Verification items for the finished model (mm, model axes). Face numbers are marked on the shaded views. A direction names the side the tool comes from. Round coordinates to 2 decimals unless told otherwise and drop trailing zeros. Write each loop counter-clockwise with the first axis right and the second up, starting at its lowest first coordinate (ties: lowest second). Pieces come first, ordered by that corner, then holes. Notation, with made-up numbers: M 56,-9 L 74,-9 A24 ccw 74,12 Z; hole C 58,14.5 d10. An arc over 180 degrees is marked long. One line per item, written item: value. Start each with the question number.
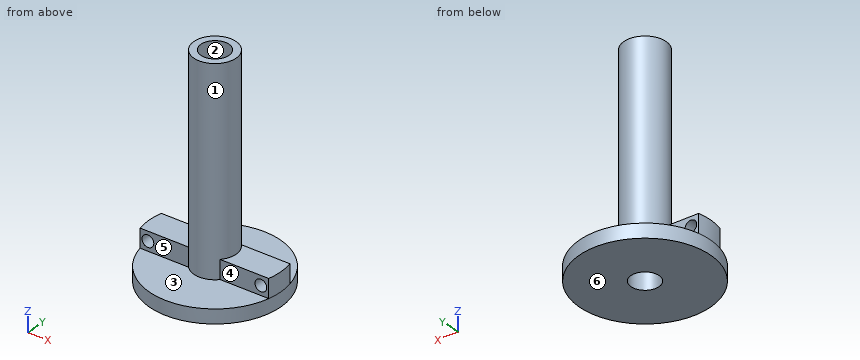
from build123d import *
from build123d.topology import SkipClean

# Parameters (mm, degrees)
SKETCH1_R           = 7
BOSS_EXTRUDE1_DEPTH = 1.5
SKETCH2_R           = 2.25
BOSS_EXTRUDE2_DEPTH = 21.5
CUT_EXTRUDE1_REACH  = 27.04
SKETCH4_R           = 1.5
BOSS_EXTRUDE5_DEPTH = 2
CUT_EXTRUDE5_REACH  = 27.5
SKETCH16_R          = 0.625
CUT_EXTRUDE6_REACH  = 25.67
SKETCH17_R          = 1.5


with BuildPart() as part:
    # Sketch1 → Boss-Extrude1 (new body)
    with BuildSketch(Plane.XY):
        Circle(SKETCH1_R)
    extrude(amount=BOSS_EXTRUDE1_DEPTH)

    # Sketch2 → Boss-Extrude2 (add)
    with BuildSketch(Plane.XY.offset(1.5)):
        Circle(SKETCH2_R)
    extrude(amount=BOSS_EXTRUDE2_DEPTH)

    # Sketch4 → Cut-Extrude1 (cut, up to next)
    with BuildSketch(Plane(origin=(0, 0, 0), x_dir=(-1, 0, 0), z_dir=(0, 0, -1)), mode=Mode.PRIVATE) as cut_extrude1_sk1:
        Circle(SKETCH4_R)
    cut_extrude1_tool1 = extrude(cut_extrude1_sk1.sketch, amount=-CUT_EXTRUDE1_REACH, mode=Mode.PRIVATE) & part.part
    add(cut_extrude1_tool1.solids().sort_by_distance((0, 0, 0))[0], mode=Mode.SUBTRACT)

    # Sketch15 → Boss-Extrude5 (add)
    with SkipClean():  # the faces are left unmerged after this step: merging them gives an invalid solid
        with BuildSketch(Plane.XY.offset(1.5)):
            with BuildLine():
                Line((6.837397, -1.5), (-6.837397, -1.5))
                ThreePointArc((-6.837397, -1.5), (-7, 0), (-6.837397, 1.5))
                Line((-6.837397, 1.5), (6.837397, 1.5))
                ThreePointArc((6.837397, 1.5), (7, 0), (6.837397, -1.5))
            make_face()
        extrude(amount=BOSS_EXTRUDE5_DEPTH)

    # Sketch16 → Cut-Extrude5 (cut, up to next)
    with BuildSketch(Plane.XZ.offset(1.5), mode=Mode.PRIVATE) as cut_extrude5_sk1:
        with Locations((-6, 2.5)):
            Circle(SKETCH16_R)
    cut_extrude5_tool1 = extrude(cut_extrude5_sk1.sketch, amount=-CUT_EXTRUDE5_REACH, mode=Mode.PRIVATE) & part.part
    # Sketch16 → Cut-Extrude5 (cut, up to next)
    with BuildSketch(Plane.XZ.offset(1.5), mode=Mode.PRIVATE) as cut_extrude5_sk2:
        with Locations(Location((6, 2.5, 0), (0, 0, 270))):
            Circle(SKETCH16_R)
    cut_extrude5_tool2 = extrude(cut_extrude5_sk2.sketch, amount=-CUT_EXTRUDE5_REACH, mode=Mode.PRIVATE) & part.part
    add(cut_extrude5_tool1.solids().sort_by_distance((-6, -1.5, 2.5))[0], mode=Mode.SUBTRACT)
    add(cut_extrude5_tool2.solids().sort_by_distance((6, -1.5, 2.5))[0], mode=Mode.SUBTRACT)

    # Sketch17 → Cut-Extrude6 (cut, up to next)
    with BuildSketch(Plane(origin=(0, 0, 1.5), x_dir=(-1, 0, 0), z_dir=(0, 0, -1)), mode=Mode.PRIVATE) as cut_extrude6_sk1:
        Circle(SKETCH17_R)
    cut_extrude6_tool1 = extrude(cut_extrude6_sk1.sketch, amount=-CUT_EXTRUDE6_REACH, mode=Mode.PRIVATE) & part.part
    add(cut_extrude6_tool1.solids().sort_by_distance((0, 0, 1.5))[0], mode=Mode.SUBTRACT)


solid = part.part
1) Thickness scan on line 1 (X direction, y = -0.5, z = 2) (3 decimals); line 2 (Y direction, x = 0, z = 14); line 3 (Z direction, x = -6, y = -0.9) (3 decimals). Record the ranges inside material, lowest first.
2) Mould release check, pull along X, two halves, no side actions. Record for the marked faces 1, 2 and 3: pulls with the +X half, pulls with the -X half, needs draft (parallel to the pull), parting line crosses it, or undercut.
3) Cross-section at D-D (z = 12.75). Record the boundary of the cut face in (x, y).
4) Gauge pin test, flat ends, axial feed: pin 1 Ø1.1 at (x, z) = (-6, 2.5) entering from -Y; pin 2 Ø1.6 at (x, z) = (3.5, 2) entering from +Y; pin 3 Ø1.5 at (x, y) = (-2.5, -5.5) entering from -Z; pin 4 Ø3.5 at (x, y) = (-5, 0) entering from +Z. Record the tip position at first contact, or that the pin passes through.
5) Cross-section at C-C (x = 0). Record the boundary of the cut face in (y, z).
6) Cross-section at B-B (z = 2.5). Record the boundary of the cut face in (x, y) (3 decimals), then the cut area to 3 significant figures.
7) Cross-section at A-A (y = 0). Record the boundary of the cut face in (x, z) (3 decimals), then the cut area to 3 significant figures.
8) Access from +Z, -Z, +X, -X, +Y, -Y to the whole of each face (thin tool, end or side, straight path). Record for the marked faces 4, 5 and 6.
Results below:
1. line 1: x = -6.982 to -6.375, -5.625 to -1.414, 1.414 to 5.625, 6.375 to 6.982
1. line 2: y = -2.25 to -1.5, 1.5 to 2.25
1. line 3: z = 0 to 1.875, 3.125 to 3.5
2. face 1: parting line crosses it
2. face 2: undercut
2. face 3: needs draft
3. outline: C 0,0 d4.5; hole C 0,0 d3
4. pin 1: passes through
4. pin 2: stops at y = 6.38
4. pin 3: stops at z = 0
4. pin 4: stops at z = 3.5
5. outline: M -7,0 L -1.5,0 L -1.5,23 L -2.25,23 L -2.25,1.5 L -7,1.5 Z; M 1.5,0 L 7,0 L 7,1.5 L 2.25,1.5 L 2.25,23 L 1.5,23 Z
6. outline: M -6.837,-1.5 L -6.625,-1.5 L -6.625,1.5 L -6.837,1.5 A7 ccw Z; M -5.375,-1.5 L -1.677,-1.5 A2.25 ccw 1.677,-1.5 L 5.375,-1.5 L 5.375,1.5 L 1.677,1.5 A2.25 ccw -1.677,1.5 L -5.375,1.5 Z; M 6.625,-1.5 L 6.837,-1.5 A7 ccw 6.837,1.5 L 6.625,1.5 Z; hole C 0,0 d3
6. area: 30.6 mm²
7. outline: M -7,0 L -1.5,0 L -1.5,23 L -2.25,23 L -2.25,3.5 L -7,3.5 Z; M 1.5,0 L 7,0 L 7,3.5 L 2.25,3.5 L 2.25,23 L 1.5,23 Z; hole C -6,2.5 d1.25; hole C 6,2.5 d1.25
7. area: 65.3 mm²
8. face 4: +Z, +X, -Y
8. face 5: +Z, -X, -Y
8. face 6: -Z, +X, -X, +Y, -Y
